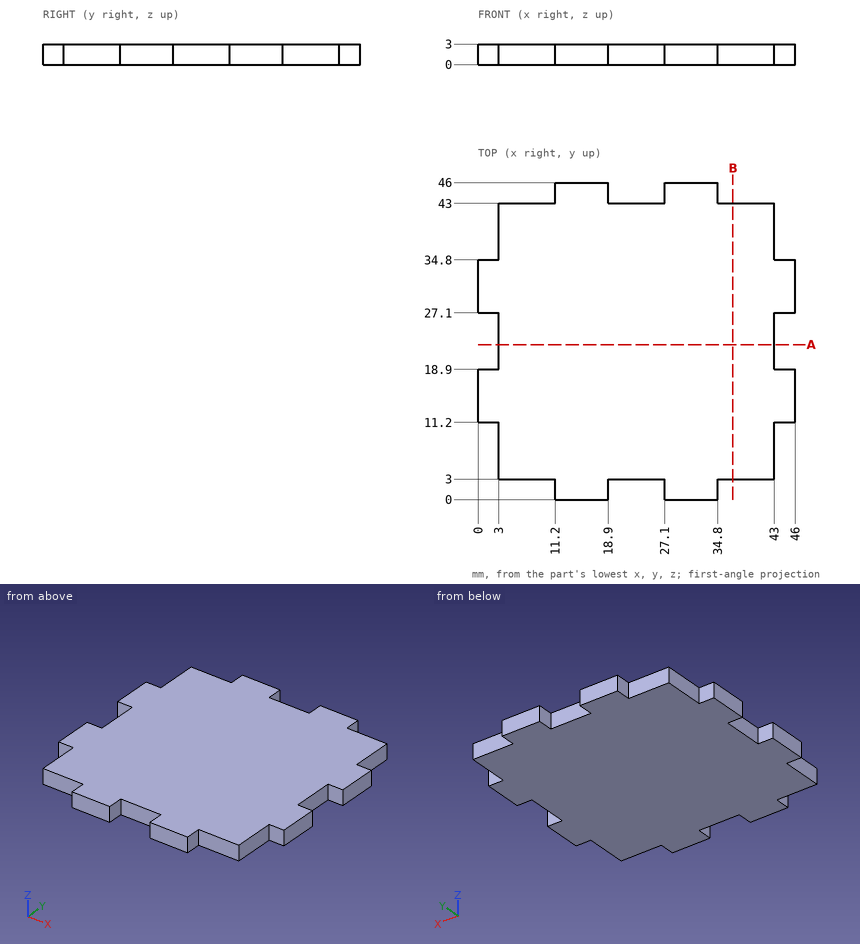
Can you work these out from the drawing? Everything is in mm from the part's minimum corner. Round coordinates to 2 decimals unless told otherwise and drop trailing zeros. Write each loop counter-clockwise with the first axis right and the second up, starting at its lowest first coordinate (ties: lowest second). Pieces come first, ordered by that corner, then holes.
1. Suppose I cut it at A-A (y = 22.5). List the corners of the cut face in (x, z) for me.
2. Will these pins go through, and if not, where does the flat tip stop? pin 1 Ø0.9 at (x, z) = (1, 1.5) entering from +Y; pin 2 Ø1.5 at (y, z) = (45, 2) entering from +X; pin 3 Ø1.5 at (x, z) = (19.5, 0.5) entering from +Y; pin 4 Ø0.9 at (y, z) = (6, 1) entering from -X.
3. I need wall thicknesses on L1, parallel to Y at x = 43.5, z = 1.75; L2, parallel to X at y = 23, z = 2.1. Which ranges of each line are inside material? Lowest first, please.
Answer sheet:
1. outline: (3, 0) - (43, 0) - (43, 3) - (3, 3) - close
2. pin 1: stops at y = 34.8
2. pin 2: stops at x = 34.8
2. pin 3: stops at y = 46
2. pin 4: stops at x = 3
3. L1: y = 11.2 to 18.9, 27.1 to 34.8
3. L2: x = 3 to 43
